Build history of the part. All positions in model axes, mm. A direction names the side the tool comes from. Give positions to 0.01 mm unless a question says otherwise; leave off trailing zeros. Loops run counter-clockwise (first coordinate to the right, second up) from the corner with the lowest first, then second, coordinate; pieces in that order, holes last. Notation, with made-up numbers: (-38.75, 24) -> (-23.75, 24) arc R36 ccw to (-23.75, 58) -> close; hole circle Ø4 at (-32, -13.5). An arc over 180 degrees is marked (long way). One line per question, with ' | ' between items. Start each with the question number.
(1) Mould opens along X. For faces 1 (the face through (-56, 2, 7.6)), 2 (the face through (87, 2, 0)), 3 (the face through (-1, 0, 14)) say: pulls with the +X half, pulls with the -X half, needs draft (parallel to the pull), parting line crosses it, or undercut.
(2) Slice it at D-D, the plane z = -26.5. Write the cut outline in (x, y), then the cut area to 3 significant figures.
(3) 3-axis set-ups, long thin cutter, end or side, ignore diameter. For faces 4 (the face through (-1, 2, 32.5)), 5 (the face through (-56, 2, -15.2)): which of +Z, -Z, +X, -X, +Y, -Y reach the whole face in a straight line?
(4) Slice it at C-C, the plane z = -7.5. Write the cut outline in (x, y).
(5) Drill centre lines: L1, parallel to Z at x = -32.5, y = 3.5; L2, parallel to Y at x = 78.5, z = 14.5; L3, parallel to Z at x = 40, y = 1.5. Where is each one in solid material? Low to high. Write a range as from..to.
(6) Slice it at B-B, the plane y = 2.5. Write the cut outline in (x, z), then the cut area to 3 significant figures.
(7) Flat gauge pin, fed straight in: pin 1 Ø3 at (x, z) = (-0.5, 20) entering from +Y. Where does the tip first touch, or does it go through?
(8) Slice it at A-A, the plane x = 56.5. Write the cut outline in (y, z).
```python
from build123d import *

# Parameters (mm, degrees)
SKETCH1_W           = 174
SKETCH1_H           = 65
BOSS_EXTRUDE1_DEPTH = 4
SKETCH2_R           = 18.25
CUT_EXTRUDE1_DEPTH  = 4
SKETCH4_W           = 50.8
SKETCH4_H           = 22.8
CUT_EXTRUDE2_DEPTH  = 4
SKETCH5_W           = 18
SKETCH5_H           = 3.531440261
CUT_EXTRUDE3_DEPTH  = 4
SKETCH9_W           = 23.248648384
SKETCH9_H           = 18.834348058
CUT_EXTRUDE4_DEPTH  = 4
SKETCH10_R          = 1.25
BOSS_EXTRUDE2_DEPTH = 3.5
SKETCH12_R          = 1.25
BOSS_EXTRUDE3_DEPTH = 3.5


with BuildPart() as part:
    # Sketch1 → Boss-Extrude1 (new body)
    with BuildSketch(Plane(origin=(0, 0, 0), x_dir=(1, 0, 0), z_dir=(0, 1, 0))):
        Rectangle(SKETCH1_W, SKETCH1_H)
    extrude(amount=BOSS_EXTRUDE1_DEPTH)

    # Sketch2 → Cut-Extrude1 (cut)
    with BuildSketch(Plane(origin=(0, 4, 0), x_dir=(1, 0, 0), z_dir=(0, 1, 0))):
        with Locations((49.293020306, 4.120013638)):
            Circle(SKETCH2_R)
    extrude(amount=-CUT_EXTRUDE1_DEPTH, mode=Mode.SUBTRACT)

    # Sketch4 → Cut-Extrude2 (cut)
    with BuildSketch(Plane(origin=(0, 4, 0), x_dir=(1, 0, 0), z_dir=(0, 1, 0))):
        with Locations((-55.970269341, 3.8)):
            Rectangle(SKETCH4_W, SKETCH4_H)
    extrude(amount=-CUT_EXTRUDE2_DEPTH, mode=Mode.SUBTRACT)

    # Sketch5 → Cut-Extrude3 (cut)
    with BuildSketch(Plane(origin=(0, 4, 0), x_dir=(1, 0, 0), z_dir=(0, 1, 0))):
        with Locations((1.8, 21.777214942)):
            Rectangle(SKETCH5_W, SKETCH5_H)
    extrude(amount=-CUT_EXTRUDE3_DEPTH, mode=Mode.SUBTRACT)

    # Sketch9 → Cut-Extrude4 (cut)
    with BuildSketch(Plane(origin=(0, 4, 0), x_dir=(1, 0, 0), z_dir=(0, 1, 0))):
        Rectangle(SKETCH9_W, SKETCH9_H)
    extrude(amount=-CUT_EXTRUDE4_DEPTH, mode=Mode.SUBTRACT)

    # Sketch10 → Boss-Extrude2 (add)
    with BuildSketch(Plane(origin=(0, 4, 0), x_dir=(1, 0, 0), z_dir=(0, 1, 0))):
        with Locations((-85.5, 31)):
            Circle(SKETCH10_R)
        with Locations((-85.5, -31)):
            Circle(SKETCH10_R)
    extrude(amount=BOSS_EXTRUDE2_DEPTH)

    # Sketch12 → Boss-Extrude3 (add)
    with BuildSketch(Plane(origin=(0, 4, 0), x_dir=(1, 0, 0), z_dir=(0, 1, 0))):
        with Locations((85.5, 31)):
            Circle(SKETCH12_R)
        with Locations((85.5, -31)):
            Circle(SKETCH12_R)
    extrude(amount=BOSS_EXTRUDE3_DEPTH)


solid = part.part
```
Final values:
1) face 1: undercut | face 2: pulls with the +X half | face 3: needs draft
2) outline: (-87, 0) -> (87, 0) -> (87, 4) -> (-87, 4) -> close | area: 696 mm2
3) face 4: +Z, +X, -X, +Y, -Y | face 5: +Y, -Y
4) outline: (-87, 0) -> (-81.37, 0) -> (-81.37, 4) -> (-87, 4) -> close; (-30.57, 0) -> (-11.62, 0) -> (-11.62, 4) -> (-30.57, 4) -> close; (11.62, 0) -> (31.36, 0) -> (31.36, 4) -> (11.62, 4) -> close; (67.23, 0) -> (87, 0) -> (87, 4) -> (67.23, 4) -> close
5) L1: -32.5..-15.2, 7.6..32.5 | L2: 0..4 | L3: -32.5..-19.83, 11.59..32.5
6) outline: (-87, -32.5) -> (87, -32.5) -> (87, 32.5) -> (-87, 32.5) -> close; hole (-81.37, -15.2) -> (-30.57, -15.2) -> (-30.57, 7.6) -> (-81.37, 7.6) -> close; hole (-11.62, -9.42) -> (11.62, -9.42) -> (11.62, 9.42) -> (-11.62, 9.42) -> close; hole (-7.2, -23.54) -> (10.8, -23.54) -> (10.8, -20.01) -> (-7.2, -20.01) -> close; hole circle Ø36.5 at (49.29, -4.12) | area: 8,600 mm2
7) pin 1: y = 4
8) outline: (0, -32.5) -> (4, -32.5) -> (4, -20.89) -> (0, -20.89) -> close; (0, 12.65) -> (4, 12.65) -> (4, 32.5) -> (0, 32.5) -> close
